```python
from build123d import *

# Parameters (mm, degrees)
F0_W     = 6.3
F0_H     = 6.3
F1_DEPTH = 2
F3_DEPTH = 5
F4_R     = 1.9
F5_DEPTH = 0.2


with BuildPart() as f1:
    # F0 (on Top) → F1 (new body)
    with BuildSketch(Plane.XY):
        with BuildLine():
            Line((21.733175, 5.734117), (-6.903563, 5.734117))
            ThreePointArc((-6.903563, 5.734117), (-10.439097, 4.269651), (-11.903563, 0.734117))
            Line((-11.903563, 0.734117), (-11.903563, -0.734117))
            ThreePointArc((-11.903563, -0.734117), (-10.439097, -4.269651), (-6.903563, -5.734117))
            Line((-6.903563, -5.734117), (21.733175, -5.734117))
            Line((21.733175, -5.734117), (21.733175, 5.734117))
        make_face()
        with Locations((-5.085194, 0)):
            Rectangle(F0_W, F0_H, mode=Mode.SUBTRACT)
        with Locations((4.914806, 0)):
            Rectangle(F0_W, F0_H, mode=Mode.SUBTRACT)
        with Locations((14.914806, 0)):
            Rectangle(F0_W, F0_H, mode=Mode.SUBTRACT)
    extrude(amount=F1_DEPTH)

    # F2 (on face) → F3 (join)
    with BuildSketch(Plane(origin=(0, 0, 0), x_dir=(1, 0, 0), z_dir=(0, 0, -1))):
        with BuildLine():
            Line((21.733175, 5.734117), (-6.903563, 5.734117))
            ThreePointArc((-6.903563, 5.734117), (-10.439097, 4.269651), (-11.903563, 0.734117))
            Line((-11.903563, 0.734117), (-11.903563, -0.734117))
            ThreePointArc((-11.903563, -0.734117), (-10.439097, -4.269651), (-6.903563, -5.734117))
            Line((-6.903563, -5.734117), (21.733175, -5.734117))
            Line((21.733175, -5.734117), (21.733175, -4.234117))
            Line((21.733175, -4.234117), (-5.403563, -4.234117))
            Line((-5.403563, -4.234117), (-6.638798, -4.234117))
            ThreePointArc((-6.638798, -4.234117), (-9.290064, -3.307969), (-10.413563, -0.734117))
            Line((-10.413563, -0.734117), (-10.413563, 0.734117))
            ThreePointArc((-10.413563, 0.734117), (-9.385508, 3.216062), (-6.903563, 4.244117))
            Line((-6.903563, 4.244117), (-5.403563, 4.244117))
            Line((-5.403563, 4.244117), (21.733175, 4.244117))
            Line((21.733175, 4.244117), (21.733175, 5.734117))
        make_face()
    extrude(amount=F3_DEPTH)

    # F4 (on face) → F5 (join)
    with BuildSketch(Plane.XY.offset(2)):
        with BuildLine():
            ThreePointArc((-11.903563, -0.734117), (-10.439097, -4.269651), (-6.903563, -5.734117))
            Line((-6.903563, -5.734117), (21.733175, -5.734117))
            Line((21.733175, -5.734117), (21.733175, 5.734117))
            Line((21.733175, 5.734117), (-6.903563, 5.734117))
            ThreePointArc((-6.903563, 5.734117), (-10.439097, 4.269651), (-11.903563, 0.734117))
            Line((-11.903563, 0.734117), (-11.903563, -0.734117))
        make_face()
        with Locations((-5.085194, 0)):
            Circle(F4_R, mode=Mode.SUBTRACT)
        with Locations((4.914806, 0)):
            Circle(F4_R, mode=Mode.SUBTRACT)
        with Locations((14.914806, 0)):
            Circle(F4_R, mode=Mode.SUBTRACT)
    extrude(amount=F5_DEPTH)


solid = f1.part
```
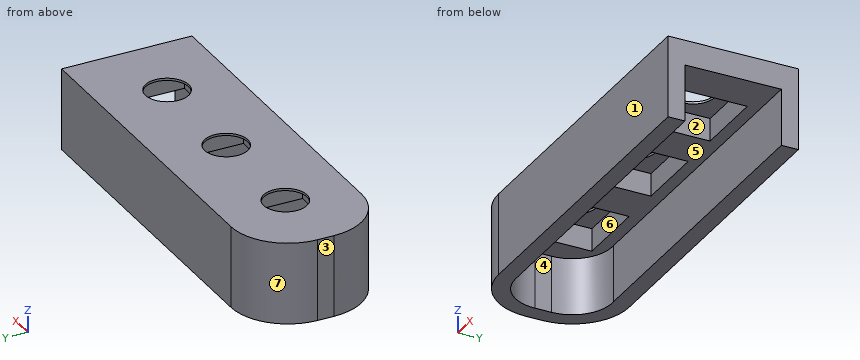
Read the model definition and answer for the solid it produces. Units are mm, in the model's axes. Face numbers are marked on the shaded views. A direction names the side the tool comes from. Give positions to 0.01 mm unless a question says otherwise; leave off trailing zeros. Order: outer loops, then holes, each group sorted by start corner. A loop starts at its lowest first (then second) coordinate and runs counter-clockwise, first axis right, second up. Notation, with made-up numbers: (34, 83.5) -> (44, 83.5) arc R35 ccw to (44, 120.5) -> close; hole circle Ø3 at (60, 55). An arc over 180 degrees is marked (long way). One line per item, written item: value. Start each with the question number.
(1) For a pull along X with two mould halves and no side action, classify the marked faces 1, 2, 3 and 4 as released by +X, released by -X, zero draft, split by the parting line, or undercut.
(2) The part is cut by section A-A (z = -1). Determine the outline of the cut face in (x, y).
(3) Straight lines are drawn through the part: L1, parallel to X at y = -0.75, z = 1; L2, parallel to Y at x = -1.5, z = -4.25; L3, parallel to Y at x = 14.5, z = 1.25. For each, find the intervals that lie inside material, in ascending order.
(4) The part is cut by section D-D (x = -10). Determine the outline of the cut face in (y, z), and give its area (3 significant figures).
(5) Flat-ended cylindrical pins translate along their axes: P1, Ø1, axis at y = -2.5, z = -3.5, coming from the -X side; P2, Ø3, axis at x = 6, y = -1, coming from the -Z side; P3, Ø0.7, axis at y = 0, z = -2, coming from the +X side. Find the tip coordinate at first contact, or state that the pin passes through.
(6) A tool of negligible diameter and unlimited length cuts with its end or side. For the marked faces 5, 6 and 7, from which of +Z, -Z, +X, -X, +Y, -Y can it reach the whole face along a straight path? Write none if from no direction.
(7) The part is cut by section B-B (y = 0). State how many separate pieces and enclosed holes the cut face has, and give its area (3 significant figures).
Taken from the geometry:
1. face 1: zero draft
1. face 2: undercut
1. face 3: released by -X
1. face 4: released by +X
2. outline: (-11.9, -0.73) arc R5 ccw to (-6.9, -5.73) -> (21.73, -5.73) -> (21.73, -4.24) -> (-6.9, -4.24) arc R3.51 cw to (-10.41, -0.73) -> (-10.41, 0.73) arc R3.51 cw to (-6.64, 4.23) -> (21.73, 4.23) -> (21.73, 5.73) -> (-6.9, 5.73) arc R5 ccw to (-11.9, 0.73) -> close
3. L1: -11.9 to -8.24, -1.94 to 1.76, 8.06 to 11.76, 18.06 to 21.73
3. L2: -5.73 to -4.24, 4.23 to 5.73
3. L3: -5.73 to -3.15, 3.15 to 5.73
4. outline: (-4.66, -5) -> (-2.39, -5) -> (-2.39, 0) -> (2.39, 0) -> (2.39, -5) -> (4.66, -5) -> (4.66, 2.2) -> (-4.66, 2.2) -> close
4. area: 43.2 mm^2
5. P1: x = -11.74
5. P2: z = 2
5. P3: x = -10.41
6. face 5: -Z, +X
6. face 6: -Z
6. face 7: +Z, -Z, -X, +Y
7. separate pieces: 4
7. enclosed holes: 0
7. area: 41.4 mm^2
